Geometry: final body of the model. Coordinates: model frame, mm. A direction names the side the tool comes from. Give positions to 0.01 mm unless a question says otherwise; leave off trailing zeros. Loops run counter-clockwise (first coordinate to the right, second up) from the corner with the lowest first, then second, coordinate; pieces in that order, holes last.
1. Section C-C, the plane y = 9.5. State how many separate pieces and enclosed holes the cut face has, then the cut area to 3 significant figures.
2. Section D-D, the plane z = -17.5. Output: boundary loops of the cut face in (x, y), then the cut area to 3 significant figures.
3. First-contact query: P1, Ø5, axis at x = -9, z = -13.5, coming from the -Y side; P2, Ø3.5, axis at y = 10, z = -17.5, coming from the -X side; P3, Ø6, axis at y = 8, z = -17, coming from the -X side; P4, Ø8, axis at x = -8, z = -14.5, coming from the +Y side. Flat tips, straight axial feed; report the tip coordinate or a pass-through.
4. Section B-B, the plane x = 10. Output: boundary loops of the cut face in (y, z), then the cut area to 3 significant figures.
5. Section A-A, the plane z = 0.5. Output: boundary loops of the cut face in (x, y).
6. Access query for faces 1 (the face through (-10.084, 16.285, -7.801)), 2 (the face through (-15, 10, -14)), 3 (the face through (-10, 4, -15)), 4 (the face through (-5, 10, -14)). Directions: +Z, -Z, +X, -X, +Y, -Y. A direction counts if a zero-diameter tool reaches every point of the face in a straight line with its end or side. Return the directions, or none.
7. Draft query along Z for faces 5 (the face through (10, 4, -15)), 6 (the face through (-15.301, 10.098, -7.785)), 7 (the face through (9.93, 10.121, -20.247)). Return one class per face: +Z half, -Z half, draft (parallel to the pull), parting line (faces both ways), or undercut.
8. Material intervals for line 1 along X through (y, z) = (-4.75, 0.5); line 2 along X through (y, z) = (12.5, -21.25); line 3 along Y through (x, z) = (-10.25, -17.5), sorted ascending.
Autodesk Inventor part; units mm, degrees
ref_plane "YZ Plane" through (0, 0, 0) normal (1, 0, 0) x (0, 1, 0)
ref_plane "XZ Plane" through (0, 0, 0) normal (0, 1, 0) x (-1, 0, 0)
ref_plane "XY Plane" through (0, 0, 0) normal (0, 0, 1) x (1, 0, 0)
sketch "Szkic2" plane through (0, 0, 0) normal (0, 1, 0) x (-1, 0, 0)
  line L0 (-20, -7.5) -> (20, -7.5)
  line L1 (20, -7.5) -> (20, 7.5)
  line L2 (20, 7.5) -> (-20, 7.5)
  line L3 (-20, 7.5) -> (-20, -7.5)
  line L4 (-20, -7.5) -> (20, 7.5) construction
  line L5 (20, -7.5) -> (-20, 7.5) construction
  point P0 (0, 0)
  dimension "d12" = 40
  dimension "d13" = 15
extrude "Wyciągnięcie proste1" add sketch "Szkic2" along normal mid plane 20
sketch "Szkic3" plane through (0, 10, 0) normal (0, 1, 0) x (1, 0, 0)
  line L0 (18, 7.5) -> (-18, 7.5)
  line L1 (-18, 7.5) -> (-18, -7.5)
  line L2 (-18, -7.5) -> (18, -7.5)
  line L3 (18, -7.5) -> (18, 7.5)
  line L4 (18, 7.5) -> (-18, -7.5) construction
  line L5 (-18, 7.5) -> (18, -7.5) construction
  circle A0 centre (10, -0.5) radius 6
  circle A1 centre (-10, -0.5) radius 6
  circle A2 centre (10, -0.5) radius 3.7
  circle A3 centre (-10, -0.5) radius 3.7
  line L6 (-20, -7.5) -> (20, -7.5)
  point P0 (0, 0)
  point P1 (10, -7)
  point P2 (10, 8)
  point P3 (-13.3166, 8)
  point P4 (-10, -7)
  point P5 (15.1962, -4)
  point P6 (-15.1962, -4)
  dimension "d16" = 36
  dimension "d17" = 15
  dimension "d18" = 12
  dimension "d19" = 8
  dimension "d20" = 8
  dimension "d21" = 12
  dimension "d22" = 8
  dimension "d23" = 8
  dimension "d24" = 7.4
  dimension "d25" = 7.4
fillet "Zaokrąglenie1" radius 2 4 edges at (20, 0, 7.5) (-20, 0, 7.5) (20, 0, -7.5) (-20, 0, -7.5)
extrude "Wyciągnięcie proste3" add sketch "Szkic3" along normal blind 20 contours L3 L2 L1 L0 | A0 | A1
sketch "Szkic4" plane through (18, 10, -7.5) normal (0, 0, -1) x (-1, 0, 0)
  line L0 (33, 0) -> (23, -20) construction
  line L1 (23, 0) -> (33, -20) construction
  line L2 (13, 6) -> (3, 6)
  line L3 (3, 6) -> (3, -6)
  line L4 (3, -6) -> (13, -6)
  line L5 (13, -6) -> (13, 6)
  line L6 (13, 6) -> (3, -6) construction
  line L7 (3, 6) -> (13, -6) construction
  line L8 (36, -20) -> (0, -20)
  line L9 (0, 0) -> (36, 0)
  line L10 (-2, 0) -> (-2, -20)
  line L11 (0, 20) -> (36, 20)
  point P0 (18, -10)
  point P1 (28, -10)
  point P2 (8, 0)
  dimension "d32" = 14
  dimension "d38" = 10
  dimension "d39" = 5
  dimension "d68" = 14
extrude "Wyciągnięcie proste4" add sketch "Szkic4" along normal blind 15
sketch "Szkic7" plane through (5, 4, -7.5) normal (-1, 0, 0) x (0, 0, 1)
  line L0 (-15, 12) -> (-15, 0)
  line L1 (-15, 0) -> (-15, 3)
  line L2 (0, -14) -> (0, 6)
  line L3 (0, 0) -> (-15, 0)
  line L4 (0, 0) -> (-15, 0)
  line L5 (-15, 12) -> (-15, 9)
  line L6 (0, 12) -> (-15, 12)
  line L7 (0, 12) -> (-15, 12)
  circle A0 centre (-10, 6) radius 2.75
  point P0 (7.5, -4)
  dimension "d48" = 5.5
  dimension "d49" = 6
  dimension "d69" = 5
extrude "Wyciągnięcie proste6" cut sketch "Szkic7" against normal blind 15
mirror "Odbij1" about plane through (0, 0, 0) normal (1, 0, 0) of "Wyciągnięcie proste6", "Wyciągnięcie proste4"
sketch "Szkic11" plane through (0, 10, 0) normal (0, 1, 0) x (1, 0, 0)
  line L0 (18, -7.5) -> (-18, -7.5)
  line L1 (18, -7.5) -> (20, -7.5)
  line L2 (20, -7.5) -> (20, 7.5)
  line L3 (20, 7.5) -> (18, 7.5)
  line L4 (18, 7.5) -> (18, -7.5)
  point P0 (0, 0)
  dimension "d63" = 2
  dimension "d64" = 15
extrude "Wyciągnięcie proste7" cut sketch "Szkic11" against normal blind 20
mirror "Odbij3" about plane through (0, 0, 0) normal (1, 0, 0) of "Wyciągnięcie proste7"
fillet "Zaokrąglenie4" radius 2 4 edges at (-18, 10, 7.5) (-18, 10, -7.5) (18, 10, -7.5) (18, 10, 7.5)
fillet "Zaokrąglenie5" radius 1 4 edges at (-10, 16, -22.5) (-10, 4, -22.5) (10, 4, -22.5) (10, 16, -22.5)
fillet "Zaokrąglenie6" radius 1 8 edges at (-15, 10, -7.5) (-10, 16, -7.5) (-10, 4, -7.5) (-5, 10, -7.5) (10, 4, -7.5) (5, 10, -7.5) (15, 10, -7.5) (10, 16, -7.5)
sketch "Szkic12" plane through (10, 10, 0.5) normal (0, 1, 0) x (1, 0, 0)
  circle A0 centre (0, 0) radius 3.7
  point P0 (-10, 0.5)
extrude "Wyciągnięcie proste8" cut sketch "Szkic12" against normal blind 44
mirror "Odbij4" about plane through (0, 0, 0) normal (1, 0, 0) of "Wyciągnięcie proste8"
properties part number "zaslepka"
Answers below:
1. separate pieces: 3
1. enclosed holes: 2
1. area: 643 mm2
2. outline: (-15, 4) - (-5, 4) - (-5, 7.25) - (-15, 7.25) - close; (-15, 12.75) - (-5, 12.75) - (-5, 16) - (-15, 16) - close; (5, 4) - (15, 4) - (15, 7.25) - (5, 7.25) - close; (5, 12.75) - (15, 12.75) - (15, 16) - (5, 16) - close
2. area: 130 mm2
3. P1: stops at y = 4
3. P2: passes through
3. P3: stops at x = -15
3. P4: stops at y = 16
4. outline: (-10, -7.5) - (3, -7.5) arc R1 cw to (4, -8.5) - (4, -21.5) arc R1 ccw to (5, -22.5) - (15, -22.5) arc R1 ccw to (16, -21.5) - (16, -8.5) arc R1 cw to (17, -7.5) - (30, -7.5) - (30, -3.2) - (-10, -3.2) - close; (-10, 4.2) - (30, 4.2) - (30, 7.5) - (-10, 7.5) - close; hole circle Ø5.5 at (10, -17.5)
4. area: 460 mm2
5. outline: (-18, -10) - (-13.7, -10) - (-13.7, 30) - (-18, 30) - close; (-6.3, -10) - (6.3, -10) - (6.3, 30) - (-6.3, 30) - close; (13.7, -10) - (18, -10) - (18, 30) - (13.7, 30) - close
6. face 1: -Z, +X, -X, +Y
6. face 2: -Z, -X, +Y, -Y
6. face 3: -Z, +X, -X, -Y
6. face 4: -Z, +Y, -Y
7. face 5: draft
7. face 6: -Z half
7. face 7: undercut
8. line 1: x = -18 to -13.7, -6.3 to 6.3, 13.7 to 18
8. line 2: x = -15 to -5, 5 to 15
8. line 3: y = 4 to 7.25, 12.75 to 16
